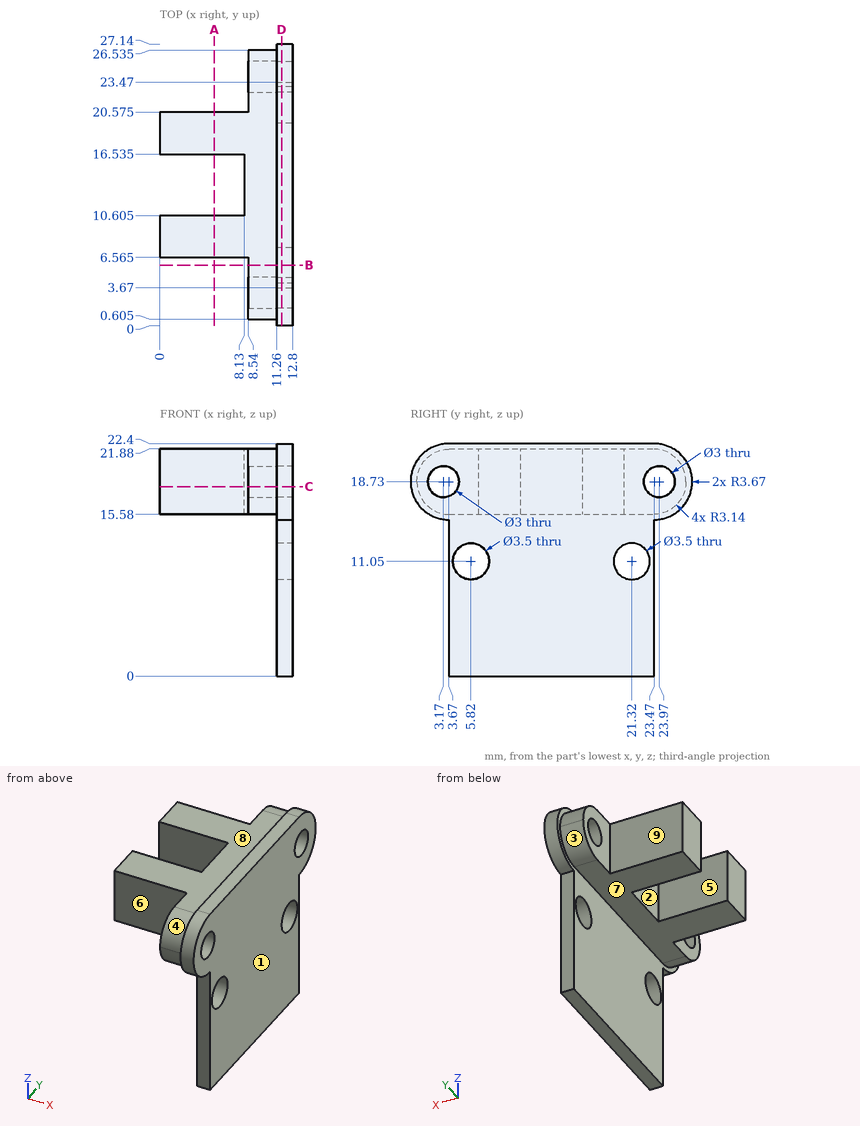
Here's the drawing with two shaded views (mm, measured from the low corner). I have some questions. A direction names the side the tool comes from. Round coordinates to 2 decimals unless told otherwise and drop trailing zeros. Loops run counter-clockwise (first coordinate to the right, second up) from the corner with the lowest first, then second, coordinate; pieces in that order, holes last.
Item 1: Suppose I cut it at D-D, the plane x = 11.75. Write out the boundary of the cut face in (y, z), then the cut area to 3 significant figures.
Item 2: Please list where these lines run through material, in increasing order: L1, parallel to X at y = 16, z = 6.25; L2, parallel to Z at x = 12.2, y = 21.32; L3, parallel to X at y = 11.75, z = 20.
Item 3: Suppose I cut it at C-C, the plane z = 18.25. Write out the boundary of the cut face in (x, y) (3 decimals), then the cut area to 3 significant figures.
Item 4: If we mould it in two halves opening along Y, with no side actions, what happens to the marked faces 1, 2, 3 and 4? For each: +Y half, -Y half, draft (parallel to the pull), parting line (faces both ways), or undercut.
Item 5: Suppose I cut it at B-B, the plane y = 5.82. Write out the boundary of the cut face in (x, z).
Item 6: Will these pins go through, and if not, where does the flat tip stop? pin 1 Ø3.5 at (x, y) = (8, 17) entering from +Z; pin 2 Ø1.2 at (x, z) = (12, 7) entering from +Y; pin 3 Ø6.5 at (y, z) = (13.5, 17.5) entering from -X; pin 4 Ø6.5 at (y, z) = (24, 19) entering from -X.
Item 7: Suppose I cut it at A-A, the plane x = 5.25. Write out the boundary of the cut face in (y, z) (3 decimals).
Item 8: Which directions (+Z, -Z, +X, -X, +Y, -Y) give clear straight access to the entire face, cutting with the end or side of a thin tool? Please do the marked faces 5, 6, 7, 8 and 9.
Reported:
1. outline: (3.67, 0) - (23.47, 0) - (23.47, 15.06) arc R3.67 ccw to (23.47, 22.4) - (3.67, 22.4) arc R3.67 ccw to (3.67, 15.06) - close; hole circle Ø3 at (3.17, 18.73); hole circle Ø3.5 at (5.82, 11.05); hole circle Ø3.5 at (21.32, 11.05); hole circle Ø3 at (23.97, 18.73)
1. area: 452 mm2
2. L1: x = 11.26 to 12.8
2. L2: z = 0 to 9.3, 12.8 to 22.4
2. L3: x = 8.13 to 12.8
3. outline: (0, 6.565) - (8.54, 6.565) - (8.54, 4.591) - (12.8, 4.591) - (12.8, 22.549) - (8.54, 22.549) - (8.54, 20.575) - (0, 20.575) - (0, 16.535) - (8.13, 16.535) - (8.13, 10.605) - (0, 10.605) - close; (8.54, 0.64) - (11.26, 0.64) - (11.26, 0.032) - (12.8, 0.032) - (12.8, 1.749) - (8.54, 1.749) - close; (8.54, 25.391) - (12.8, 25.391) - (12.8, 27.108) - (11.26, 27.108) - (11.26, 26.5) - (8.54, 26.5) - close
3. area: 159 mm2
4. face 1: draft
4. face 2: undercut
4. face 3: +Y half
4. face 4: -Y half
5. outline: (8.54, 15.58) - (11.26, 15.58) - (11.26, 12.8) - (12.8, 12.8) - (12.8, 22.4) - (11.26, 22.4) - (11.26, 21.88) - (8.54, 21.88) - close; (11.26, 0) - (12.8, 0) - (12.8, 9.3) - (11.26, 9.3) - close
6. pin 1: stops at z = 21.88
6. pin 2: stops at y = 23.47
6. pin 3: stops at x = 0
6. pin 4: stops at x = 8.54
7. outline: (6.565, 15.58) - (10.605, 15.58) - (10.605, 21.88) - (6.565, 21.88) - close; (16.535, 15.58) - (20.575, 15.58) - (20.575, 21.88) - (16.535, 21.88) - close
8. face 5: +Z, -Z, -X
8. face 6: +Z, -Z, -X, -Y
8. face 7: -Z, -X, +Y, -Y
8. face 8: +Z, -X, +Y, -Y
8. face 9: +Z, -Z, -X, +Y
